Can you work these out from the model? Positions are in its coordinate system, mm. Coordinates: 2 decimals unless noted, no trailing zeros. Write each loop counter-clockwise with the first axis right and the second up, starting at its lowest first coordinate (ties: lowest second). Pieces come first, ordered by that corner, then holes. Notation, with made-up numbers: (22.5, 55) - (49.5, 55) arc R38 cw to (49.5, 94) - close; hole circle Ø5 at (47.5, 73.5). An arc over 180 degrees is marked (long way). Use one line per item in the form item = value. Start each with the question number.
(1) If we section it at B-B on y = 41.5: Please give me the cut outline in (x, z), then the cut area to 3 significant figures.
(2) If I drill on probe 1 along X at (y, z) = (-17.5, 8.25); probe 2 along X at (y, z) = (-14, 4); probe 3 along X at (y, z) = (-25.5, 14), over which ranges is the centre line in solid material (lowest first)? Write a range as from..to.
(3) For pin 1 Ø3 at (x, z) = (27, 9) entering from -Y; pin 2 Ø2 at (x, z) = (26, 13) entering from +Y; pin 3 Ø1 at (y, z) = (28.5, 12) entering from -X, each with a flat end and sliding along its axis, tell me the tip position at first contact or that it passes through.
(4) If we section it at D-D on z = 13.25: Give the number of separate pieces and of enclosed holes in the cut face, then the cut area to 3 significant figures.
(5) Thinking about a two-plate mould opening in Y: for faces 1 (the face through (-19.514, -14.715, 12.325)), 2 (the face through (7, -10, 25)), 3 (the face through (-44.534, -25.15, 12.325)), 4 (the face through (-16.75, 9.94, 12.32)), which applies, pulls with the +Y half, pulls with the -Y half, needs draft (parallel to the pull), parting line crosses it, or undercut?
(6) If we section it at A-A on x = -4: Please give me the cut outline in (y, z), then the cut area to 3 significant figures.
(7) If we section it at C-C on x = 26: Please give me the cut outline in (y, z), then the cut area to 3 significant figures.
```python
from build123d import *

# Parameters (mm, degrees)
F1_DEPTH = 7
F2_DEPTH = 25


with BuildPart() as f1:
    # F0 (on Top) → F1 (new body)
    with BuildSketch(Plane.XY):
        with BuildLine():
            ThreePointArc((41.460889, -17.5), (33.196721, -6.729927), (20.654706, -11.925))
            ThreePointArc((20.654706, -11.925), (27.425057, -28.270073), (41.460889, -17.5))
        make_face()
        with BuildLine():
            ThreePointArc((0, 11.15), (7.884241, 7.884241), (11.15, 0))
            ThreePointArc((11.15, 0), (10.770073, -2.885832), (9.656183, -5.575))
            ThreePointArc((9.656183, -5.575), (5.575, -9.656183), (0, -11.15))
            Line((0, -11.15), (0, -19.476393))
            ThreePointArc((0, -19.476393), (8.359284, -20.824585), (15.870867, -24.732445))
            ThreePointArc((15.870867, -24.732445), (44.297199, -25.575), (29.354359, -1.378351))
            ThreePointArc((29.354359, -1.378351), (16.867051, 9.738196), (13.483492, 26.110797))
            ThreePointArc((13.483492, 26.110797), (14.219408, 42.657084), (0, 51.15))
            Line((0, 51.15), (0, 46.15))
            ThreePointArc((0, 46.15), (7.884241, 42.884241), (11.15, 35))
            ThreePointArc((11.15, 35), (7.884241, 27.115759), (0, 23.85))
            Line((0, 23.85), (0, 11.15))
        make_face()
        with BuildLine():
            ThreePointArc((41.460889, -17.5), (27.425057, -28.270073), (20.654706, -11.925))
            ThreePointArc((20.654706, -11.925), (33.196721, -6.729927), (41.460889, -17.5))
        make_face(mode=Mode.SUBTRACT)
        with BuildLine():
            ThreePointArc((-19.160889, -17.5), (-19.504592, -14.752919), (-20.514513, -12.175198))
            ThreePointArc((-20.514513, -12.175198), (-41.117186, -20.247081), (-19.160889, -17.5))
        make_face()
        with BuildLine():
            ThreePointArc((-9.334502, -6.098325), (-9.80609, 5.306891), (0, 11.15))
            Line((0, 11.15), (0, 23.85))
            ThreePointArc((0, 23.85), (-11.15, 35), (0, 46.15))
            Line((0, 46.15), (0, 51.15))
            ThreePointArc((0, 51.15), (-14.219408, 42.657084), (-13.483492, 26.110797))
            ThreePointArc((-13.483492, 26.110797), (-16.867051, 9.738196), (-29.354359, -1.378351))
            ThreePointArc((-29.354359, -1.378351), (-44.297199, -25.575), (-15.870867, -24.732445))
            ThreePointArc((-15.870867, -24.732445), (-8.359284, -20.824585), (0, -19.476393))
            Line((0, -19.476393), (0, -11.15))
            ThreePointArc((0, -11.15), (-5.306891, -9.80609), (-9.334502, -6.098325))
        make_face()
        with BuildLine():
            ThreePointArc((-19.160889, -17.5), (-41.117186, -20.247081), (-20.514513, -12.175198))
            ThreePointArc((-20.514513, -12.175198), (-19.504592, -14.752919), (-19.160889, -17.5))
        make_face(mode=Mode.SUBTRACT)
    extrude(amount=F1_DEPTH)

    # F0 (on Top) → F2 (join)
    with BuildSketch(Plane.XY):
        with BuildLine():
            ThreePointArc((41.460889, -17.5), (33.196721, -6.729927), (20.654706, -11.925))
            ThreePointArc((20.654706, -11.925), (27.425057, -28.270073), (41.460889, -17.5))
        make_face()
        with BuildLine():
            ThreePointArc((0, 11.15), (7.884241, 7.884241), (11.15, 0))
            ThreePointArc((11.15, 0), (10.770073, -2.885832), (9.656183, -5.575))
            ThreePointArc((9.656183, -5.575), (5.575, -9.656183), (0, -11.15))
            Line((0, -11.15), (0, -19.476393))
            ThreePointArc((0, -19.476393), (8.359284, -20.824585), (15.870867, -24.732445))
            ThreePointArc((15.870867, -24.732445), (44.297199, -25.575), (29.354359, -1.378351))
            ThreePointArc((29.354359, -1.378351), (16.867051, 9.738196), (13.483492, 26.110797))
            ThreePointArc((13.483492, 26.110797), (14.219408, 42.657084), (0, 51.15))
            Line((0, 51.15), (0, 46.15))
            ThreePointArc((0, 46.15), (7.884241, 42.884241), (11.15, 35))
            ThreePointArc((11.15, 35), (7.884241, 27.115759), (0, 23.85))
            Line((0, 23.85), (0, 11.15))
        make_face()
        with BuildLine():
            ThreePointArc((41.460889, -17.5), (27.425057, -28.270073), (20.654706, -11.925))
            ThreePointArc((20.654706, -11.925), (33.196721, -6.729927), (41.460889, -17.5))
        make_face(mode=Mode.SUBTRACT)
        with BuildLine():
            ThreePointArc((-19.160889, -17.5), (-19.504592, -14.752919), (-20.514513, -12.175198))
            ThreePointArc((-20.514513, -12.175198), (-41.117186, -20.247081), (-19.160889, -17.5))
        make_face()
        with BuildLine():
            ThreePointArc((-9.334502, -6.098325), (-9.80609, 5.306891), (0, 11.15))
            Line((0, 11.15), (0, 23.85))
            ThreePointArc((0, 23.85), (-11.15, 35), (0, 46.15))
            Line((0, 46.15), (0, 51.15))
            ThreePointArc((0, 51.15), (-14.219408, 42.657084), (-13.483492, 26.110797))
            ThreePointArc((-13.483492, 26.110797), (-16.867051, 9.738196), (-29.354359, -1.378351))
            ThreePointArc((-29.354359, -1.378351), (-44.297199, -25.575), (-15.870867, -24.732445))
            ThreePointArc((-15.870867, -24.732445), (-8.359284, -20.824585), (0, -19.476393))
            Line((0, -19.476393), (0, -11.15))
            ThreePointArc((0, -11.15), (-5.306891, -9.80609), (-9.334502, -6.098325))
        make_face()
        with BuildLine():
            ThreePointArc((-19.160889, -17.5), (-41.117186, -20.247081), (-20.514513, -12.175198))
            ThreePointArc((-20.514513, -12.175198), (-19.504592, -14.752919), (-19.160889, -17.5))
        make_face(mode=Mode.SUBTRACT)
    extrude(amount=F2_DEPTH)


solid = f1.part
```
Reported:
q1.outline = (-14.78, 0) - (-9.06, 0) - (-9.06, 25) - (-14.78, 25) - close; (9.06, 0) - (14.78, 0) - (14.78, 25) - (9.06, 25) - close
q1.area = 286 mm2
q2.probe_1 = -46.46..-41.46, -19.16..19.16, 41.46..46.46
q2.probe_2 = -46.08..-40.9, -19.72..19.72, 40.9..46.08
q2.probe_3 = -44.34..-38.08, -22.54..-16.28, 16.28..22.54, 38.08..44.34
q3.pin_1 = -33.55
q3.pin_2 = 1.01
q3.pin_3 = -14.99
q4.separate_pieces = 1
q4.enclosed_holes = 4
q4.area = 2,380 mm2
q5.face_1 = undercut
q5.face_2 = needs draft
q5.face_3 = parting line crosses it
q5.face_4 = undercut
q6.outline = (-19.78, 0) - (-10.41, 0) - (-10.41, 25) - (-19.78, 25) - close; (10.41, 0) - (24.59, 0) - (24.59, 25) - (10.41, 25) - close; (45.41, 0) - (50.65, 0) - (50.65, 25) - (45.41, 25) - close
q6.area = 720 mm2
q7.outline = (-33.06, 0) - (-27.78, 0) - (-27.78, 25) - (-33.06, 25) - close; (-7.22, 0) - (0.36, 0) - (0.36, 25) - (-7.22, 25) - close
q7.area = 322 mm2
